Study the drawing (mm; zero at the part's minimum x, y, z) and answer. Coordinates: 2 decimals unless noted, no trailing zeros. Loops run counter-clockwise (first coordinate to the right, second up) from the corner with the lowest first, then second, coordinate; pieces in that order, holes last. Notation, with made-up numbers: (26.5, 11.5) - (37.5, 11.5) arc R23 cw to (37.5, 46.5) - close; hole circle Ø1 at (-20.5, -1.75). An arc over 180 degrees is marked (long way). Use CSV: the item, a comma, the result in double quotes.
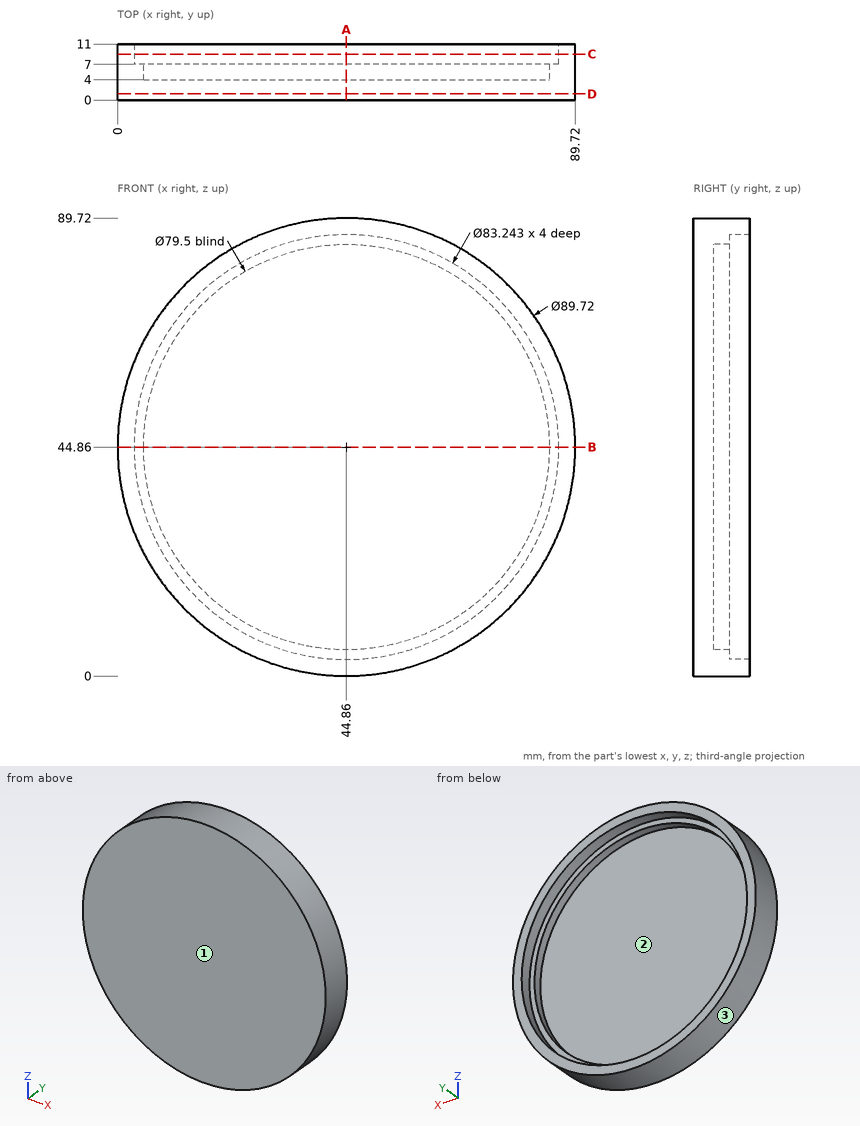
Q1. The part is cut by section C-C on y = 9. Determine the outline of the cut face in (x, z).
Reported:
outline,"circle Ø89.72 at (44.86, 44.86); hole circle Ø83.24 at (44.86, 44.86)"
Q2. The part is cut by section B-B on z = 44.86. Determine the outline of the cut face in (x, y).
Reported:
outline,"(0, 0) - (89.72, 0) - (89.72, 11) - (86.48, 11) - (86.48, 7) - (84.61, 7) - (84.61, 4) - (5.11, 4) - (5.11, 7) - (3.24, 7) - (3.24, 11) - (0, 11) - close"
Q3. For a pull along Z with two mould halves and no side action, classify the marked faces 1, 2 and 3 as +Z half, -Z half, draft (parallel to the pull), parting line (faces both ways), or undercut.
Reported:
face 1,"draft"
face 2,"undercut"
face 3,"parting line"
Q4. The part is cut by section D-D on y = 1.25. Determine the outline of the cut face in (x, z).
Reported:
outline,"circle Ø89.72 at (44.86, 44.86)"
Q5. The part is cut by section A-A on x = 44.86. Determine the outline of the cut face in (y, z).
Reported:
outline,"(0, 0) - (11, 0) - (11, 3.24) - (7, 3.24) - (7, 5.11) - (4, 5.11) - (4, 84.61) - (7, 84.61) - (7, 86.48) - (11, 86.48) - (11, 89.72) - (0, 89.72) - close"
Q6. Given P1, Ø2, axis at x = 73.5, y = 8.5, coming from the +Z side; P2, Ø2, axis at x = 19.5, y = 6, coming from the +Z side; P3, Ø5, axis at y = 9, z = 25.5, coming from the +X side; P4, Ø6, axis at x = 63.5, z = 72, coming from the -Y side, each flat-ended and moving along its own axis, determine where each tip first touches the part or whether it passes through.
Reported:
P1,"stops at z = 80.19"
P2,"stops at z = 82.53"
P3,"stops at x = 86.43"
P4,"stops at y = 0"
Q7. Find the intervals of material crossed by probe 1 along X at (y, z) = (5.75, 44); probe 2 along Y at (x, z) = (22.5, 74); probe 3 along Z at (x, y) = (73.5, 6.75) (1 decimal), in increasing order. Write a range as [from, to].
Reported:
probe 1,"x = [0.01, 5.12], [84.6, 89.71]"
probe 2,"y = [0, 4]"
probe 3,"z = [10.3, 17.3], [72.4, 79.4]"
